from build123d import *

# Parameters (mm, degrees)
SKETCH_1_W      = 90
SKETCH_1_H      = 65
EXTRUDE_1_DEPTH = 5
HOLE_WIZARD_1_D = 5.5
HOLE_WIZARD_2_D = 5.5
CHAMFER_1_SIZE  = 1.80208992
CHAMFER_2_SIZE  = 1.80208992
FILLET_1_R      = 5
FILLET_2_R      = 5


with BuildPart() as part:
    # 草图1 → 凸台-拉伸1 (new body)
    with BuildSketch(Plane(origin=(0, 0, 0), x_dir=(-1, 0, 0), z_dir=(0, 0, -1))):
        with Locations((0, 72.5)):
            Rectangle(SKETCH_1_W, SKETCH_1_H)
    extrude(amount=-EXTRUDE_1_DEPTH)

    # 孔1 (through all)
    with Locations(Plane.XY.offset(5)):
        with Locations((-20, 85)):
            Hole(HOLE_WIZARD_1_D / 2)

    # 孔2 (through all)
    with Locations(Plane.XY.offset(5)):
        with Locations((20, 85)):
            Hole(HOLE_WIZARD_2_D / 2)

    # 倒角1
    chamfer_1_edges = [part.edges().sort_by_distance(p)[0] for p in [
        (-17.25, 85, 5),
    ]]
    chamfer(chamfer_1_edges, length=CHAMFER_1_SIZE)

    # 倒角2
    chamfer_2_edges = [part.edges().sort_by_distance(p)[0] for p in [
        (22.75, 85, 5),
    ]]
    chamfer(chamfer_2_edges, length=CHAMFER_2_SIZE)

    # 圆角1
    fillet_1_edges = [part.edges().sort_by_distance(p)[0] for p in [
        (45, 105, 2.5),
    ]]
    fillet(fillet_1_edges, radius=FILLET_1_R)

    # 圆角2
    fillet_2_edges = [part.edges().sort_by_distance(p)[0] for p in [
        (-45, 105, 2.5),
    ]]
    fillet(fillet_2_edges, radius=FILLET_2_R)


solid = part.part
The listing builds one solid part. Answer for the finished solid, in the listing's coordinates (mm). Round coordinates to 2 decimals unless told otherwise and drop trailing zeros. Write each loop counter-clockwise with the first axis right and the second up, starting at its lowest first coordinate (ties: lowest second). Pieces come first, ordered by that corner, then holes. Notation, with made-up numbers: M 58,0 L 107,0 A12 ccw 107,23 Z; hole C -6,45.25 d8. An arc over 180 degrees is marked long. Write each question's results on one line, items separated by ' | '. Start each with the question number.
(1) This flat-tipped pin is pushed along its axis until it touches: P1, Ø5, axis at x = 20, y = 85, coming from the -Z side. Where does it stop, or does it pass through?
(2) Determine the mould class of faces 1 (the flat face through (1, 105, 2)), 2 (the flat face through (45, 70, 2)), 3 (the cylindrical face through (-17.253, 85.121, 1.577)) for opening direction Y: +Y half, -Y half, draft (parallel to the pull), parting line (faces both ways), or undercut.
(3) The part is cut by section A-A, the plane y = 85. Write down the section's boundary in (x, z), and give its area (3 significant figures).
(4) Find the intervals of material crossed by line 1 (Y direction, x = -20, z = 1.75); line 2 (X direction, y = 101.5, z = 2.25); line 3 (X direction, y = 102, z = 1.75), in increasing order.
(5) The part is cut by section B-B, the plane x = -20. Write down the section's boundary in (y, z), and give its area (3 significant figures).
Worked answers:
1) P1: passes through
2) face 1: +Y half | face 2: draft | face 3: undercut
3) outline: M -45,0 L -22.75,0 L -22.75,3.2 L -24.55,5 L -45,5 Z; M -17.25,0 L 17.25,0 L 17.25,3.2 L 15.45,5 L -15.45,5 L -17.25,3.2 Z; M 22.75,0 L 45,0 L 45,5 L 24.55,5 L 22.75,3.2 Z | area: 389 mm²
4) line 1: y = 40 to 82.25, 87.75 to 105 | line 2: x = -44.77 to 44.77 | line 3: x = -44.58 to 44.58
5) outline: M 40,0 L 82.25,0 L 82.25,3.2 L 80.45,5 L 40,5 Z; M 87.75,0 L 105,0 L 105,5 L 89.55,5 L 87.75,3.2 Z | area: 294 mm²
